Input: part model. Units: mm. Frame: model coordinates. Face numbers are marked on the shaded views. A direction names the side the tool comes from. Give positions to 0.01 mm unless a question says otherwise; leave off trailing zeros. Loops run counter-clockwise (first coordinate to the right, second up) from the corner with the lowest first, then second, coordinate; pieces in that order, holes last. Notation, with made-up numbers: (51.5, -30) - (102.5, -30) arc R19 ccw to (102.5, -18) - close; hole circle Ø10 at (8.5, -27.5). An arc over 180 degrees is marked (long way). Answer as a JSON object with one key per item and string values. Group by question number.
(1) Access query for the marked faces 1, 2 and 3. Directions: +Z, -Z, +X, -X, +Y, -Y. A direction counts if a zero-diameter tool reaches every point of the face in a straight line with its end or side. Return the directions, or none.
(2) Mould query, pull axis Y, two halves, no side actions, for the marked faces 4, 5 and 6. Classes: +Y half, -Y half, draft (parallel to the pull), parting line (faces both ways), or undercut.
(3) Section query B-B (y = 20.5). Return loops of the section in (x, z).
(4) Pin query (flat end, axial travel): P1, Ø10, axis at x = -85, z = -4.5, coming from the +Y side; P2, Ø21, axis at x = 198.77, y = 481.49, coming from the +Z side; P3, Ø3, axis at x = 4, y = 47.5, coming from the -Z side; P4, Ø5, axis at x = -224, z = 22.5, coming from the +Y side. Return the tip coordinate at first contact, or that it passes through.
(5) Section query C-C (x = 395.5). Return loops of the section in (y, z), plus the area to 3 significant figures.
(6) Section query D-D (y = 301.5). Return loops of the section in (x, z).
(7) Material intervals for L1, parallel to X at y = -235, z = -17; L2, parallel to Z at x = -4.5, y = 349.5; L3, parallel to Z at x = -38, y = 227.5, sorted ascending.
(8) Section query A-A (x = 262.5). Return loops of the section in (y, z).
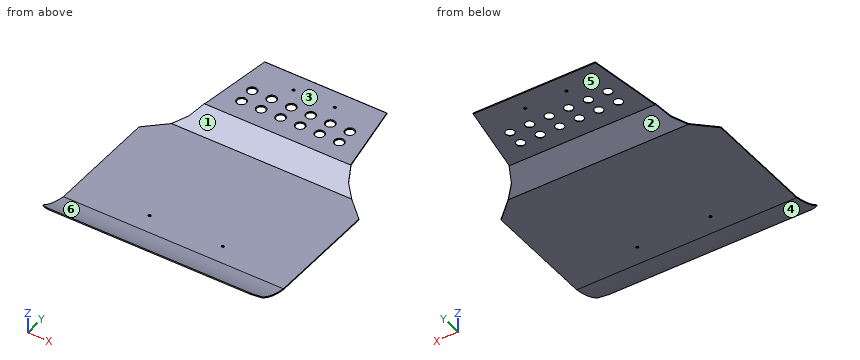
```python
from build123d import *

# Parameters (mm, degrees)
F2_DEPTH        = 450
F5_DEPTH        = 137
F7_DEPTH        = 134.9001572951
F9_D            = 11
F12_D           = 11
F14_D           = 35
F14_CSINK_D     = 40
F14_CSINK_ANGLE = 90


with BuildPart() as f2:
    # F1 (on offset) → F2 (new body, through all)
    with BuildSketch(Plane.YZ.offset(450)):
        with BuildLine():
            ThreePointArc((633.4541976452, 15.1353164322), (635.4541972499, 17.135316037), (633.4541976452, 19.1353156418))
            Line((633.4541976452, 19.1353156418), (333.4541976452, 19.1353156418))
            Line((333.4541976452, 19.1353156418), (233.4541976452, -30.8646843582))
            Line((233.4541976452, -30.8646843582), (-316.5458023548, -10.8646843582))
            ThreePointArc((-316.5458023548, -10.8646843582), (-395.7263494601, 14.2619563044), (-466.5458023548, 57.6844412928))
            ThreePointArc((-466.5458023548, 57.6844412928), (-468.6915325534, 56.8348647408), (-469.0341345652, 54.5526372621))
            ThreePointArc((-469.0341345652, 54.5526372621), (-397.2522499905, 10.5614235075), (-316.9897726189, -14.8511829484))
            Line((-316.9897726189, -14.8511829484), (234.329521914, -34.8991572951))
            Line((234.329521914, -34.8991572951), (334.3984693686, 15.1353164322))
            Line((334.3984693686, 15.1353164322), (633.4541976452, 15.1353164322))
        make_face()
    extrude(amount=-F2_DEPTH)

    # F4 (on offset) → F5 (cut)
    with BuildSketch(Plane.XY.offset(100)):
        Polygon((498.5155965069, 703.4857805286), (218.7778259494, 735.3884513889), (237.0079512575, 712.9704888378), (297.9584336281, 337.6117348671), (326.3231515884, 278.4070670605), (368.6494827271, 233.5909307003), (451.0919357517, 153.3712233816), (483.6110378483, 153.3712233816), align=None)
    extrude(amount=-F5_DEPTH, mode=Mode.SUBTRACT)

    # F6 (on offset) → F7 (cut, through all)
    with BuildSketch(Plane.XY.offset(100)):
        with BuildLine():
            ThreePointArc((478.8447916508, -417.378693819), (427.8834958855, -460.3781245943), (367.9305016994, -489.5610511303))
            Line((367.9305016994, -489.5610511303), (478.8447916508, -496.6032207012))
            Line((478.8447916508, -496.6032207012), (478.8447916508, -417.378693819))
        make_face()
    extrude(amount=-F7_DEPTH, mode=Mode.SUBTRACT)

    # F9 (through all)
    with Locations(Plane.XY.offset(19.1353156418)):
        with Locations((84.2372775078, 561.8938207626)):
            Hole(F9_D / 2)

    # F10: F2 across plane


with BuildPart() as f2_1:
    add(f2.part)
    add(f2.part.mirror(Plane.YZ))

    # F12 (through all)
    with Locations(Plane(origin=(0, -0.8125779098, -22.3458925199), x_dir=(1, 0, 0), z_dir=(0, 0.0363396181, 0.9993394979))):
        with Locations((-150, -236.43194139), (150, -236.43194139)):
            Hole(F12_D / 2)

    # F14 (through all)
    with Locations(Plane.XY.offset(19.1353156418)):
        with Locations((198.7729519606, 481.4921915531), (118.7729519606, 481.4921915531), (38.7729519606, 481.4921915531), (-41.2270480394, 481.4921915531), (-121.2270480394, 481.4921915531), (-201.2270480394, 481.4921915531), (-201.2270480394, 415.4921915531), (-121.2270480394, 415.4921915531), (-41.2270480394, 415.4921915531), (38.7729519606, 415.4921915531), (118.7729519606, 415.4921915531), (198.7729519606, 415.4921915531)):
            CounterSinkHole(F14_D / 2, F14_CSINK_D / 2, counter_sink_angle=F14_CSINK_ANGLE)


solid = f2_1.part
```
Recorded:
{
 "1": {"face 1": "+Z, +X, -X", "face 2": "-Z, +X, -X, +Y", "face 3": "+Z, +X, -X, +Y"},
 "2": {"face 4": "-Y half", "face 5": "draft", "face 6": "undercut"},
 "3": {"outline": "(-450, -27.12) - (450, -27.12) - (450, -23.12) - (-450, -23.12) - close"},
 "4": {"P1": "stops at y = 305.13", "P2": "passes through", "P3": "stops at z = -28.16", "P4": "stops at y = -407.67"},
 "5": {"outline": "(-469.03, 54.55) arc R347.06 ccw to (-316.99, -14.85) - (207.46, -33.92) - (207.46, -29.92) - (-316.55, -10.86) arc R343.06 cw to (-466.55, 57.68) arc R2.31 ccw to start", "area": "2,770 mm^2"},
 "6": {"outline": "(-315.26, -1.31) - (315.26, -1.31) - (315.26, 3.16) - (-315.26, 3.16) - close"},
 "7": {"L1": "x = -450 to -155.04, -144.96 to 144.96, 155.04 to 450", "L2": "z = 15.14 to 19.14", "L3": "z = -34.65 to -30.65"},
 "8": {"outline": "(-469.03, 54.55) arc R347.06 ccw to (-316.99, -14.85) - (234.33, -34.9) - (334.4, 15.14) - (555.98, 15.14) - (555.98, 19.14) - (333.45, 19.14) - (233.45, -30.86) - (-316.55, -10.86) arc R343.06 cw to (-466.55, 57.68) arc R2.31 ccw to start"}
}
